Check sheet for the modelled part. Datum: model origin and axes. Units: mm. Coordinates: 2 decimals unless noted, no trailing zeros. Loops run counter-clockwise (first coordinate to the right, second up) from the corner with the lowest first, then second, coordinate; pieces in that order, holes last. Notation, with made-up numbers: (-35.5, 69.5) - (13.5, 69.5) arc R33 cw to (13.5, 106.5) - close; hole circle Ø5 at (61.5, -22). An arc over 180 degrees is marked (long way). Write each question's results on one line, items separated by ' | '. Start each with the question number.
1. Thickness scan on line 1 (Y direction, x = 1.25, z = -15.6); line 2 (Z direction, x = 2, y = 70); line 3 (Y direction, x = 2.75, z = 14). Record the ranges inside material, lowest first. Write a range as [from, to].
2. Draft check along Y on faces 1 (the face through (1.48, 78.59, -16.17)), 2 (the face through (0, -1, -15)). Enter one of: released by +Y, released by -Y, zero draft, split by the parting line, or undercut.
3. Cross-section at A-A (x = 2.05). Give the number of separate pieces and of enclosed holes in the cut face, and give its area (3 significant figures).
4. Cross-section at B-B (y = 70). Record the cut outline in (x, z), and give its area (3 significant figures).
5. Gauge pin test, flat ends, axial feed: P1, Ø12, axis at y = -28.5, z = 18, coming from the -X side; P2, Ø10, axis at y = 0, z = 0, coming from the -X side. Record the tip position at first contact, or that the pin passes through.
6. Cross-section at C-C (z = 15). Record the cut outline in (x, y).
```python
from build123d import *

# Parameters (mm, degrees)
SKETCH1_W           = 200
SKETCH1_H           = 70
SKETCH1_R           = 8.5
SKETCH1_R_2         = 2.65
SKETCH1_W_2         = 20
SKETCH1_H_2         = 3
BOSS_EXTRUDE1_DEPTH = 3


with BuildPart() as part:
    # Sketch1 → Boss-Extrude1 (new body)
    with BuildSketch(Plane.YZ):
        Rectangle(SKETCH1_W, SKETCH1_H)
        with Locations(Location((0, 0, 0), (0, 0, 270))):
            Circle(SKETCH1_R, mode=Mode.SUBTRACT)
        with Locations(Location((-76, -15.6, 0), (0, 0, 270))):
            Circle(SKETCH1_R_2, mode=Mode.SUBTRACT)
        with Locations(Location((76, -15.6, 0), (0, 0, 90))):
            Circle(SKETCH1_R_2, mode=Mode.SUBTRACT)
        with Locations(Location((-70, 15, 0), (0, 0, 270))):
            Circle(SKETCH1_R_2, mode=Mode.SUBTRACT)
        with Locations(Location((70, 15, 0), (0, 0, 90))):
            Circle(SKETCH1_R_2, mode=Mode.SUBTRACT)
        with Locations((-70, -26.5)):
            Rectangle(SKETCH1_W_2, SKETCH1_H_2, mode=Mode.SUBTRACT)
        with Locations((70, -26.5)):
            Rectangle(SKETCH1_W_2, SKETCH1_H_2, mode=Mode.SUBTRACT)
        with Locations((0, -26.5)):
            Rectangle(SKETCH1_W_2, SKETCH1_H_2, mode=Mode.SUBTRACT)
        with Locations((70, 26.5)):
            Rectangle(SKETCH1_W_2, SKETCH1_H_2, mode=Mode.SUBTRACT)
        with Locations((0, 26.5)):
            Rectangle(SKETCH1_W_2, SKETCH1_H_2, mode=Mode.SUBTRACT)
        with Locations((-70, 26.5)):
            Rectangle(SKETCH1_W_2, SKETCH1_H_2, mode=Mode.SUBTRACT)
    extrude(amount=BOSS_EXTRUDE1_DEPTH)


solid = part.part
```
Established:
1) line 1: [-100, -78.65], [-73.35, 73.35], [78.65, 100] | line 2: [-35, -28], [-25, 12.35], [17.65, 25], [28, 35] | line 3: [-100, -72.45], [-67.55, 67.55], [72.45, 100]
2) face 1: undercut | face 2: zero draft
3) separate pieces: 1 | enclosed holes: 11 | area: 13,300 mm^2
4) outline: (0, -35) - (3, -35) - (3, -28) - (0, -28) - close; (0, -25) - (3, -25) - (3, 12.35) - (0, 12.35) - close; (0, 17.65) - (3, 17.65) - (3, 25) - (0, 25) - close; (0, 28) - (3, 28) - (3, 35) - (0, 35) - close | area: 176 mm^2
5) P1: x = 0 | P2: through
6) outline: (0, -100) - (3, -100) - (3, -72.65) - (0, -72.65) - close; (0, -67.35) - (3, -67.35) - (3, 67.35) - (0, 67.35) - close; (0, 72.65) - (3, 72.65) - (3, 100) - (0, 100) - close
